Autodesk Inventor part; units mm, degrees
ref_plane "YZ Plane" through (0, 0, 0) normal (1, 0, 0) x (0, 1, 0)
ref_plane "XZ Plane" through (0, 0, 0) normal (0, 1, 0) x (-1, 0, 0)
ref_plane "XY Plane" through (0, 0, 0) normal (0, 0, 1) x (1, 0, 0)
sketch "Sketch1" plane through (0, 0, 0) normal (0, 0, 1) x (1, 0, 0)
  line L0 (0, 12.6249) -> (38.1, 12.6249)
  line L1 (38.1, 12.6249) -> (38.1, 7.8624)
  line L2 (38.1, 7.8624) -> (4.7625, 7.8624)
  line L3 (4.7625, 7.8624) -> (4.7625, -25.4751)
  line L4 (4.7625, -25.4751) -> (0, -25.4751)
  line L5 (0, -25.4751) -> (0, 12.6249)
  point P0 (0, 0)
  point P1 (0, 0)
  dimension "d0" = 38.1
  dimension "d1" = 4.7625
  dimension "d2" = 4.7625
  dimension "d3" = 38.1
extrude "Extrusion1" add sketch "Sketch1" along normal blind 76.2
fillet "Corner Round1" radius 50.8 1 edges at (38.1, 10.2436, 0)
equation "\"BendRadius\" = Thickness"
equation "\"BendReliefWidth\" = Thickness"
equation "\"BendReliefDepth\" = 0.5 * Thickness"
equation "\"CornerReliefSize\" = 4 * Thickness"
equation "\"MinimumRemnant\" = 2 * Thickness"
equation "\"TransitionRadius\" = BendRadius"
equation "\"JacobiRadiusSize\" = BendRadius"
equation "\"GapSize\" = Thickness"
properties part number "RearWheelMountLeft" material "Steel, Mild"
For this review, take the finished solid that the model builds, in its own axes (mm). A direction names the side the tool comes from. Give positions to 0.01 mm unless a question says otherwise; leave off trailing zeros. Write each loop counter-clockwise with the first axis right and the second up, starting at its lowest first coordinate (ties: lowest second). Pieces come first, ordered by that corner, then holes.
Item 1: Take a section at D-D (z = 52.5). Give the boundary of the cut face in (x, y).
Item 2: Take a section at C-C (x = 30.5). Give the boundary of the cut face in (y, z), and give its area (3 significant figures).
Item 3: Insertion check: P1, Ø5, axis at x = 15, z = 9, coming from the -Y side; P2, Ø2, axis at y = -16.5, z = 65, coming from the +X side; P3, Ø2, axis at y = -10, z = 52, coming from the -X side. Each pin has a flat end and moves straight along its axis. Give the tip position at first contact, or say it passes through.
Item 4: Take a section at A-A (z = 34.5). Give the boundary of the cut face in (x, y).
Item 5: Machinability: for faces 1 (the face through (4.762, -9, 38)), 2 (the face through (38.1, 10, 63)), which of the approach directions +Z, -Z, +X, -X, +Y, -Y give a long, thin tool a straight path to every point of the face, cutting with its end or side? Answer none if there is none.
Item 6: Wall thickness on probe 1 along Y at (x, z) = (25, 55); probe 2 along X at (y, z) = (-2, 14.5); probe 3 along Z at (x, y) = (13, 11): over which ranges is each line inside the solid? List them lowest first.
Item 7: Take a section at B-B (y = 6). Give the boundary of the cut face in (x, z), and give its area (3 significant figures).
Established:
1. outline: (0, -25.48) - (4.76, -25.48) - (4.76, 7.86) - (38.1, 7.86) - (38.1, 12.62) - (0, 12.62) - close
2. outline: (7.86, 22.46) - (12.62, 22.46) - (12.62, 76.2) - (7.86, 76.2) - close
2. area: 256 mm2
3. P1: stops at y = 7.86
3. P2: stops at x = 4.76
3. P3: stops at x = 0
4. outline: (0, -25.48) - (4.76, -25.48) - (4.76, 7.86) - (35.93, 7.86) - (35.93, 12.62) - (0, 12.62) - close
5. face 1: +Z, -Z, +X, -Y
5. face 2: +Z, -Z, +X, +Y, -Y
6. probe 1: y = 7.86 to 12.62
6. probe 2: x = 0 to 4.76
6. probe 3: z = 5.37 to 76.2
7. outline: (0, 0) arc R50.8 ccw to (4.76, 1.48) - (4.76, 76.2) - (0, 76.2) - close
7. area: 360 mm2
